```python
from build123d import *

# Parameters (mm, degrees)
BOSS_EXTRUDE1_DEPTH = 37
FILLET1_R           = 3
SKETCH2_R           = 1.5
SKETCH2_W           = 19.44
SKETCH2_H           = 3.5
CUT_EXTRUDE1_DEPTH  = 49.745330033
SKETCH3_R           = 2.7
BOSS_EXTRUDE2_DEPTH = 21


with BuildPart() as part:
    # Sketch1 → Boss-Extrude1 (new body)
    with BuildSketch(Plane(origin=(0, 0, 0), x_dir=(1, 0, 0), z_dir=(0, 1, 0))):
        Polygon((0, 0), (22.44, 0), (22.44, 3), (3, 3), (3, 22.44), (0, 22.44), align=None)
    extrude(amount=BOSS_EXTRUDE1_DEPTH)

    # Fillet1
    fillet1_edges = [part.edges().sort_by_distance(p)[0] for p in [
        (3, 18.5, -3),
    ]]
    fillet(fillet1_edges, radius=FILLET1_R)

    # Sketch2 → Cut-Extrude1 (cut, through all)
    with BuildSketch(Plane(origin=(0, 0, -22.44), x_dir=(-1, 0, 0), z_dir=(0, 0, -1))):
        with Locations((-11.212785563, 27.75)):
            Circle(SKETCH2_R)
        with Locations((-17.212785563, 18.5)):
            Circle(SKETCH2_R)
        with Locations((-11.212785563, 9.25)):
            Circle(SKETCH2_R)
        with Locations((-12.72, 1.75)):
            Rectangle(SKETCH2_W, SKETCH2_H)
        with Locations((-12.72, 35.25)):
            Rectangle(SKETCH2_W, SKETCH2_H)
    extrude(amount=-CUT_EXTRUDE1_DEPTH, mode=Mode.SUBTRACT)

    # Sketch3 → Boss-Extrude2 (add)
    with BuildSketch(Plane.ZY):
        with Locations(Location((-11.22, 11, 0), (0, 0, 180))):
            Circle(SKETCH3_R)
    extrude(amount=BOSS_EXTRUDE2_DEPTH)


solid = part.part
```
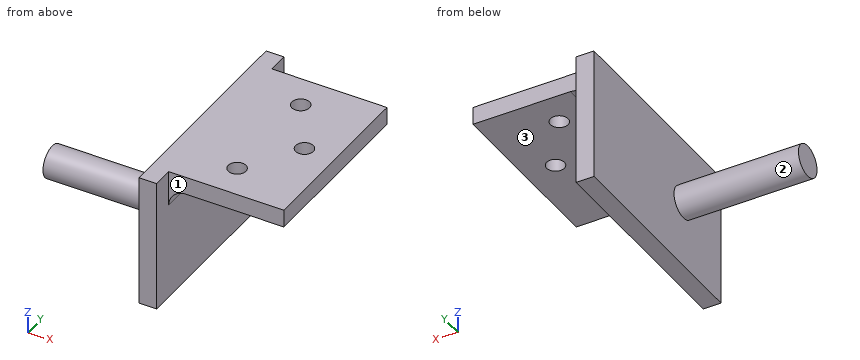
Input: part model. Units: mm. Frame: model coordinates. Face numbers are marked on the shaded views. A direction names the side the tool comes from. Give positions to 0.01 mm unless a question says otherwise; leave off trailing zeros. Order: outer loops, then holes, each group sorted by start corner. A loop starts at its lowest first (then second) coordinate and runs counter-clockwise, first axis right, second up. Notation, with made-up numbers: (59, 48) -> (102, 48) arc R31 cw to (102, 80) -> close; hole circle Ø2 at (-13, 4). An arc over 180 degrees is marked (long way). Write each question's results on one line, items separated by ' | '. Start each with the question number.
Item 1: Line query: line 1 (Z direction, x = 7.5, y = 6.5); line 2 (X direction, y = 12, z = -20.75); line 3 (Z direction, x = -5, y = 12). Output: solid intervals per line, ascending.
Item 2: Set-up query: the marked faces 1, 2 and 3. Return all of +Z, -Z, +X, -X, +Y, -Y with unobstructed straight access to the full face (end or side cutting, diameter ignored); none if empty.
Item 3: Cut plane C-C on x = 17.5. Return the cut outline in (y, z).
Item 4: Cut plane D-D on y = 22. Return the cut outline in (x, z).
Item 5: Contact query for flat-ended pins moving along their axis: P1, Ø12, axis at x = -15.5, z = -11, coming from the -Y side; P2, Ø3, axis at x = 9, z = -2, coming from the -Y side; P3, Ø12, axis at y = 14, z = -17, coming from the +X side; P4, Ø2.5, axis at x = 17.21, y = 18.5, coming from the -Z side. Output: stop coordinate, or through.
Item 6: Cut plane B-B on z = -11.22. Return the cut outline in (x, y).
Item 7: Cut plane A-A on y = 27.75. Return the cut outline in (x, z).
Established:
1) line 1: -3 to 0 | line 2: 0 to 3 | line 3: -13.73 to -8.71
2) face 1: +Z, -Z, +X, -Y | face 2: -X | face 3: -Z, +X, +Y, -Y
3) outline: (3.5, -3) -> (17.03, -3) -> (17.03, 0) -> (3.5, 0) -> close; (19.97, -3) -> (33.5, -3) -> (33.5, 0) -> (19.97, 0) -> close
4) outline: (0, -22.44) -> (3, -22.44) -> (3, -6) arc R3 cw to (6, -3) -> (22.44, -3) -> (22.44, 0) -> (0, 0) -> close
5) P1: y = 8.3 | P2: y = 3.5 | P3: x = 3 | P4: through
6) outline: (-21, 8.3) -> (0, 8.3) -> (0, 0) -> (3, 0) -> (3, 37) -> (0, 37) -> (0, 13.7) -> (-21, 13.7) -> close
7) outline: (0, -22.44) -> (3, -22.44) -> (3, -6) arc R3 cw to (6, -3) -> (9.71, -3) -> (9.71, 0) -> (0, 0) -> close; (12.71, -3) -> (22.44, -3) -> (22.44, 0) -> (12.71, 0) -> close
